The listing builds one solid part. Answer for the finished solid, in the listing's coordinates (mm). A direction names the side the tool comes from. Round coordinates to 2 decimals unless told otherwise and drop trailing zeros. Order: outer loops, then holes, each group sorted by start corner. A loop starts at its lowest first (then second) coordinate and runs counter-clockwise, first axis right, second up. Notation, with made-up numbers: (61.5, -21) - (65.5, -21) arc R25 cw to (65.5, 12) - close; hole circle Ø9 at (18, 35.5). An arc over 180 degrees is marked (long way). Use CSV: the item, a comma, the result in double quotes. Start each with the question number.
Item 1: Straight lines are drawn through the part: line 1 along X through (y, z) = (0, 7.5); line 2 along Z through (x, y) = (12.5, 15); line 3 along X through (y, z) = (4.5, 4.25). For each, find the intervals that lie inside material, in ascending order. Write a range as [from, to].
Item 2: Find section B-B, the plane y = 0. Give the vertices of the cut face in (x, z), plus the area to 3 significant figures.
Item 3: Find section A-A, the plane x = 0. Give the vertices of the cut face in (y, z).
Item 4: For faces 1 (the flat face through (2, 9, 7)), 2 (the flat face through (0, 17, 0)), 3 (the cylindrical face through (12.932, -5.362, 16.77)), determine the directions among +Z, -Z, +X, -X, +Y, -Y from which every point of the face is accessible in a straight line to the end or side of a thin tool.
Item 5: Flat-ended cylindrical pins translate along their axes: P1, Ø1.6, axis at y = 9, z = 11, coming from the -X side (3 decimals); P2, Ø4, axis at x = 12, z = 7.5, coming from the +Y side; P3, Ø2, axis at y = 21.5, z = 3.5, coming from the -X side; P4, Ø3, axis at x = 1, z = 11.5, coming from the -Y side. Find the tip coordinate at first contact, or state that the pin passes through.
Item 6: Determine the mould class of faces 4 (the flat face through (0, 17, 14.4)), 5 (the cylindrical face through (0, 28, 7)), 6 (the flat face through (0, 9.8, 7)) for opening direction X: +X half, -X half, draft (parallel to the pull), parting line (faces both ways), or undercut.
```python
from build123d import *

# Parameters (mm, degrees)
CAMBODY_DEPTH   = 14.4
BOSS_DEPTH      = 2.75
BOSS_DEPTH_BACK = 17.25
SKETCH2_R       = 14
BOSSFILLETS_R   = 2
SKETCH3_R       = 8
BORE_DEPTH      = 40.799497605
SKETCH4_W       = 4
SKETCH4_H       = 5
KEYSLOT_DEPTH   = 40.799497605


with BuildPart() as part:
    # Sketch1 → CamBody (new body)
    with BuildSketch(Plane.XY):
        with BuildLine():
            ThreePointArc((8, 24), (0, 28), (-8, 24))
            add(Edge.make_bspline(
                [(-8, 24), (-9.885763615, 21.485648513), (-14.768346923, 15.874245369), (-18.297603119, 9.133687845), (-19.364916731, 5)],
                knots=[0, 0, 0, 0, 0.425985114, 1, 1, 1, 1], degree=3))
            ThreePointArc((-19.364916731, 5), (0, -20), (19.364916731, 5))
            add(Edge.make_bspline(
                [(19.364916731, 5), (18.228780394, 9.400237112), (14.835269856, 16.032711081), (9.974620681, 21.367172425), (8, 24)],
                knots=[0, 0, 0, 0, 0.579854245, 1, 1, 1, 1], degree=3))
        make_face()
    extrude(amount=CAMBODY_DEPTH)

    # Sketch2 → Boss (add, two sides: drawn at the far end of the back side and taken through both)
    with BuildSketch(Plane.XY.offset(14.4).offset(-BOSS_DEPTH_BACK)):
        Circle(SKETCH2_R)
    extrude(amount=BOSS_DEPTH + BOSS_DEPTH_BACK)

    # BossFillets
    bossfillets_edges = [part.edges().sort_by_distance(p)[0] for p in [
        (-14, 0, 0),
        (-14, 0, 14.4),
    ]]
    fillet(bossfillets_edges, radius=BOSSFILLETS_R)

    # Sketch3 → Bore (cut, through all)
    with BuildSketch(Plane.XY.offset(17.15)):
        Circle(SKETCH3_R)
    extrude(amount=-BORE_DEPTH, mode=Mode.SUBTRACT)

    # Sketch4 → KeySlot (cut, through all)
    with BuildSketch(Plane.XY.offset(17.15)):
        with Locations((0, 7.3)):
            Rectangle(SKETCH4_W, SKETCH4_H)
    extrude(amount=-KEYSLOT_DEPTH, mode=Mode.SUBTRACT)


solid = part.part
```
Worked out:
1,line 1,"x = [-20, -8], [8, 20]"
1,line 2,"z = [0, 14.4]"
1,line 3,"x = [-19.49, -6.61], [6.61, 19.49]"
2,outline,"(-20, 0) - (-16, 0) arc R2 cw to (-14, -2) - (-14, -2.85) - (-8, -2.85) - (-8, 17.15) - (-14, 17.15) - (-14, 16.4) arc R2 cw to (-16, 14.4) - (-20, 14.4) - close; (8, -2.85) - (14, -2.85) - (14, -2) arc R2 cw to (16, 0) - (20, 0) - (20, 14.4) - (16, 14.4) arc R2 cw to (14, 16.4) - (14, 17.15) - (8, 17.15) - close"
2,area,"416 mm²"
3,outline,"(-20, 0) - (-16, 0) arc R2 cw to (-14, -2) - (-14, -2.85) - (-8, -2.85) - (-8, 17.15) - (-14, 17.15) - (-14, 16.4) arc R2 cw to (-16, 14.4) - (-20, 14.4) - close; (9.8, -2.85) - (14, -2.85) - (14, -2) arc R2 cw to (16, 0) - (28, 0) - (28, 14.4) - (16, 14.4) arc R2 cw to (14, 16.4) - (14, 17.15) - (9.8, 17.15) - close"
4,face 1,"+Z, -Z"
4,face 2,"-Z"
4,face 3,"+Z"
5,P1,"stops at x = -18.335"
5,P2,"stops at y = 21.46"
5,P3,"stops at x = -10.74"
5,P4,"stops at y = -20"
6,face 4,"draft"
6,face 5,"parting line"
6,face 6,"undercut"
